The listing builds one solid part. Answer for the finished solid, in the listing's coordinates (mm). Face numbers are marked on the shaded views. A direction names the side the tool comes from. Give positions to 0.01 mm unless a question says otherwise; leave off trailing zeros. Write each loop counter-clockwise with the first axis right and the second up, starting at its lowest first coordinate (ties: lowest second). Pieces come first, ordered by that corner, then holes. Notation, with made-up numbers: (-2, 2.25) - (36, 2.25) arc R12 ccw to (36, 17.25) - close; hole circle Ø7 at (4.5, 35.5). An arc over 180 degrees is marked (long way). Use a Markdown table: item, result. Add a question column.
from build123d import *

# Parameters (mm, degrees)
ESQUISSE1_W                                      = 45
ESQUISSE1_H                                      = 29
BOSS_EXTRU_1_DEPTH                               = 14
ESQUISSE8_W                                      = 45
ESQUISSE8_H                                      = 23
BOSS_EXTRU_2_DEPTH                               = 0.01
ESQUISSE3_R                                      = 1
ESQUISSE3_R_2                                    = 0.8
ESQUISSE3_R_3                                    = 0.65
ESQUISSE3_R_4                                    = 1.25
ESQUISSE3_R_5                                    = 1.5
ENL_V_MAT_EXTRU_2_DEPTH                          = 1.01
ENL_V_MAT_EXTRU_2_DEPTH_BACK                     = 15
ESQUISSE4_W                                      = 10
ESQUISSE4_H                                      = 14
ENL_V_MAT_EXTRU_3_DEPTH                          = 46
CONG_1_R                                         = 5
CONG_2_R                                         = 2
ESQUISSE5_R                                      = 1.5
ENL_V_MAT_EXTRU_4_DEPTH                          = 13
FRAISAGE_POUR_VIS_T_TE_FRAIS_E_6_PAN_D           = 3.4
FRAISAGE_POUR_VIS_T_TE_FRAIS_E_6_PAN_CSINK_D     = 6.72
FRAISAGE_POUR_VIS_T_TE_FRAIS_E_6_PAN_CSINK_ANGLE = 90
TROU_POUR_TARAUDAGE_POUR_TROU_TARAUD_M5_D        = 4.2
TROU_POUR_TARAUDAGE_POUR_TROU_TARAUD_M5_DEPTH    = 6
TROU_POUR_TARAUDAGE_POUR_TROU_TARAUD_M5_TIP      = 1.2618073
D_GAGEMENT_M2_51_D                               = 2.9
D_GAGEMENT_M2_51_DEPTH                           = 5
D_GAGEMENT_M2_51_TIP                             = 0.871247898
CONG_4_R                                         = 2
CHANFREIN1_SIZE                                  = 4
CHANFREIN1_SIZE2                                 = 1.865
CONG_5_R                                         = 2


with BuildPart() as part:
    # Esquisse1 → Boss.-Extru.1 (new body)
    with BuildSketch(Plane.XY):
        Rectangle(ESQUISSE1_W, ESQUISSE1_H)
    extrude(amount=BOSS_EXTRU_1_DEPTH)

    # Esquisse8 → Boss.-Extru.2 (add)
    with BuildSketch(Plane.XY.offset(14)):
        with Locations((0, -3)):
            Rectangle(ESQUISSE8_W, ESQUISSE8_H)
    extrude(amount=BOSS_EXTRU_2_DEPTH)

    # Esquisse3 → Enlèv. mat.-Extru.2 (cut, two sides)
    with BuildSketch(Plane.XY.offset(14)) as enl_v_mat_extru_2_sk:
        with Locations((0, 11)):
            Circle(ESQUISSE3_R)
        with Locations((-8.5, 11)):
            Circle(ESQUISSE3_R_2)
        with Locations((-17, 11)):
            Circle(ESQUISSE3_R_3)
        with Locations((8.5, 11)):
            Circle(ESQUISSE3_R_4)
        with Locations((17, 11)):
            Circle(ESQUISSE3_R_5)
    extrude(amount=ENL_V_MAT_EXTRU_2_DEPTH, mode=Mode.SUBTRACT)
    extrude(enl_v_mat_extru_2_sk.sketch, amount=-ENL_V_MAT_EXTRU_2_DEPTH_BACK, mode=Mode.SUBTRACT)

    # Esquisse4 → Enlèv. mat.-Extru.3 (cut, through all)
    with BuildSketch(Plane.ZY.offset(22.5)):
        with Locations((5, -7.5)):
            Rectangle(ESQUISSE4_W, ESQUISSE4_H)
    extrude(amount=-ENL_V_MAT_EXTRU_3_DEPTH, mode=Mode.SUBTRACT)

    # Congé1
    cong_1_edges = [part.edges().sort_by_distance(p)[0] for p in [
        (22.5, 14.5, 7),
        (-22.5, 14.5, 7),
    ]]
    fillet(cong_1_edges, radius=CONG_1_R)

    # Congé2
    cong_2_edges = [part.edges().sort_by_distance(p)[0] for p in [
        (0, -0.5, 10),
    ]]
    fillet(cong_2_edges, radius=CONG_2_R)

    # Esquisse5 → Enlèv. mat.-Extru.4 (cut)
    with BuildSketch(Plane.XZ.offset(0.5)):
        with Locations(Location((17, 5, 0), (0, 0, 270))):  # turned: the seam where the file's is
            Circle(ESQUISSE5_R)
        with Locations(Location((8.5, 5, 0), (0, 0, 270))):  # turned: the seam where the file's is
            Circle(ESQUISSE5_R)
        with Locations(Location((0, 5, 0), (0, 0, 270))):  # turned: the seam where the file's is
            Circle(ESQUISSE5_R)
        with Locations(Location((-8.5, 5, 0), (0, 0, 270))):  # turned: the seam where the file's is
            Circle(ESQUISSE5_R)
        with Locations(Location((-17, 5, 0), (0, 0, 270))):  # turned: the seam where the file's is
            Circle(ESQUISSE5_R)
    extrude(amount=-ENL_V_MAT_EXTRU_4_DEPTH, mode=Mode.SUBTRACT)

    # Fraisage pour vis à tête fraisée à 6 pans creux M31 (through all)
    with Locations(Plane(origin=(0, 0, 10), x_dir=(-1, 0, 0), z_dir=(0, 0, -1))):
        with Locations((-13.5, -7.5), (13.5, -7.5), (0, -7.5)):
            CounterSinkHole(FRAISAGE_POUR_VIS_T_TE_FRAIS_E_6_PAN_D / 2, FRAISAGE_POUR_VIS_T_TE_FRAIS_E_6_PAN_CSINK_D / 2, counter_sink_angle=FRAISAGE_POUR_VIS_T_TE_FRAIS_E_6_PAN_CSINK_ANGLE)

    # Trou pour taraudage pour trou taraudé M51
    with Locations(Plane(origin=(0, -0.5, 0), x_dir=(-1, 0, 0), z_dir=(0, -1, 0))):
        with Locations((17, -5), (8.5, -5), (0, -5), (-8.5, -5), (-17, -5)):
            Hole(TROU_POUR_TARAUDAGE_POUR_TROU_TARAUD_M5_D / 2, depth=TROU_POUR_TARAUDAGE_POUR_TROU_TARAUD_M5_DEPTH)
            with Locations((0, 0, -(TROU_POUR_TARAUDAGE_POUR_TROU_TARAUD_M5_DEPTH + TROU_POUR_TARAUDAGE_POUR_TROU_TARAUD_M5_TIP / 2))):  # 118° drill point
                Cone(0, TROU_POUR_TARAUDAGE_POUR_TROU_TARAUD_M5_D / 2, TROU_POUR_TARAUDAGE_POUR_TROU_TARAUD_M5_TIP, mode=Mode.SUBTRACT)

    # Dégagement M2.51
    with Locations(Plane(origin=(0, 0, 0), x_dir=(-1, 0, 0), z_dir=(0, 0, -1))):
        with Locations((-12.5, 8.5), (12.5, 8.5)):
            Hole(D_GAGEMENT_M2_51_D / 2, depth=D_GAGEMENT_M2_51_DEPTH)
            with Locations((0, 0, -(D_GAGEMENT_M2_51_DEPTH + D_GAGEMENT_M2_51_TIP / 2))):  # 118° drill point
                Cone(0, D_GAGEMENT_M2_51_D / 2, D_GAGEMENT_M2_51_TIP, mode=Mode.SUBTRACT)

    # Congé4
    cong_4_edges = [part.edges().sort_by_distance(p)[0] for p in [
        (0, -0.5, 0),
    ]]
    fillet(cong_4_edges, radius=CONG_4_R)

    # Chanfrein1
    chanfrein1_edges = [part.edges().sort_by_distance(p)[0] for p in [
        (0, -14.5, 10),
    ]]
    chanfrein1_side = [part.faces().sort_by_distance(p)[0] for p in [
        (0, -14.5, 12.005),
    ]]
    chamfer(chanfrein1_edges, length=CHANFREIN1_SIZE, length2=CHANFREIN1_SIZE2, reference=chanfrein1_side[0])

    # Congé5
    cong_5_edges = [part.edges().sort_by_distance(p)[0] for p in [
        (0, -12.635, 10),
    ]]
    fillet(cong_5_edges, radius=CONG_5_R)


solid = part.part
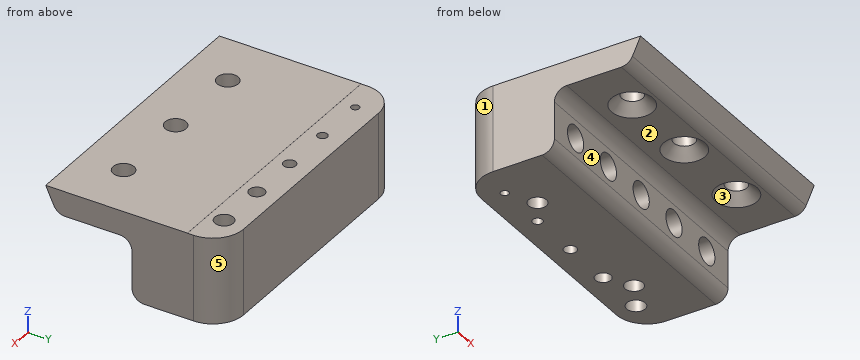
1. The part is cut by section B-B (x = -8.5). Count the separate pieces of the cut face and the enclosed holes in it, and give its area (3 significant figures).
2. Given P1, Ø5.5, axis at x = 0, y = -7.5, coming from the -Z side; P2, Ø2.5, axis at x = -3, y = -7, coming from the -Z side; P3, Ø3, axis at x = -0.5, z = 8, coming from the -Y side, each flat-ended and moving along its own axis, determine where each tip first touches the part or whether it passes through.
3. For a pull along X with two mould halves and no side action, classify the marked faces 3, 4 and 5 as released by +X, released by -X, zero draft, split by the parting line, or undercut.
4. Consider L1, parallel to Y at x = 12.5, z = 2.4; L2, parallel to Y at x = -8.5, z = 2.45; L3, parallel to X at y = 11, z = 9.5. Determine where each line is inside the solid, lowest interval first. Write a range as [from, to].
5. The part is cut by section D-D (z = 9). Give the vertices of the cut face in (x, y).
6. Which of the six approach directions +Z, -Z, +X, -X, +Y, -Y give full straight-line access (tool end or side, diameter ignored) to the marked faces 1 and 2?
7. The part is cut by section A-A (y = -7.5). Give the vertices of the cut face in (x, z), and give its area (3 significant figures).
Check values:
| question | item | result |
|---|---|---|
| 1 | separate pieces | 3 |
| 1 | enclosed holes | 0 |
| 1 | area | 198 mm2 |
| 2 | P1 | stops at z = 10.61 |
| 2 | P2 | stops at z = 10 |
| 2 | P3 | stops at y = -1.18 |
| 3 | face 3 | undercut |
| 3 | face 4 | zero draft |
| 3 | face 5 | released by +X |
| 4 | L1 | y = [-0.5, 7.05], [9.95, 14.5] |
| 4 | L2 | y = [-0.5, 10.2], [11.8, 14.5] |
| 4 | L3 | x = [-22.27, -17.65], [-16.35, -9.3], [-7.7, -1], [1, 7.25], [9.75, 15.5], [18.5, 22.27] |
| 5 | outline | (-22.5, -0.77) - (22.5, -0.77) - (22.5, 9.5) arc R5 ccw to (17.5, 14.5) - (-17.5, 14.5) arc R5 ccw to (-22.5, 9.5) - close; hole circle Ø1.3 at (-17, 11); hole circle Ø1.6 at (-8.5, 11); hole circle Ø2 at (0, 11); hole circle Ø2.5 at (8.5, 11); hole circle Ø3 at (17, 11) |
| 6 | face 1 | +Z, -Z, -X, +Y |
| 6 | face 2 | -Z, +X, -X, -Y |
| 7 | outline | (-22.5, 10) - (-16.86, 10) - (-15.2, 11.66) - (-15.2, 14.01) - (-22.5, 14.01) - close; (-11.8, 11.66) - (-10.14, 10) - (-3.36, 10) - (-1.7, 11.66) - (-1.7, 14.01) - (-11.8, 14.01) - close; (1.7, 11.66) - (3.36, 10) - (10.14, 10) - (11.8, 11.66) - (11.8, 14.01) - (1.7, 14.01) - close; (15.2, 11.66) - (16.86, 10) - (22.5, 10) - (22.5, 14.01) - (15.2, 14.01) - close |
| 7 | area | 131 mm2 |
